Here's how the part is built. I have some questions about the finished solid (model axes, mm). Round coordinates to 2 decimals unless told otherwise and drop trailing zeros. Loops run counter-clockwise (first coordinate to the right, second up) from the corner with the lowest first, then second, coordinate; pieces in that order, holes last. Notation, with made-up numbers: M 66,55.25 L 80,55.25 A29 ccw 80,80.25 Z; hole C 13.25,55.25 d11. An arc over 180 degrees is marked long. Use a Markdown table: item, result.
```python
from build123d import *

# Parameters (mm, degrees)
SKETCH1_R           = 10.922
BOSS_EXTRUDE1_DEPTH = 5.08
SKETCH4_W           = 2.413
SKETCH4_H           = 2.413


with BuildPart() as part:
    # Sketch1 → Boss-Extrude1 (new body)
    with BuildSketch(Plane(origin=(0, 0, 0), x_dir=(1, 0, 0), z_dir=(0, 1, 0))):
        with Locations(Location((0, 0, 0), (0, 0, 270))):
            Circle(SKETCH1_R)
    extrude(amount=BOSS_EXTRUDE1_DEPTH)

    # Sketch4 → Cut-Revolve1 (revolve, cut)
    with BuildSketch(Plane.XY, mode=Mode.PRIVATE) as cut_revolve1_sk:
        with Locations((10.8077, 2.4765)):
            Rectangle(SKETCH4_W, SKETCH4_H)
    revolve(cut_revolve1_sk.sketch.rotate(Axis((0, 0, 0), (0, 1, 0)), 90), axis=Axis((0, 0, 0), (0, 1, 0)), mode=Mode.SUBTRACT)

    # Sketch5 → Revolve1 (revolve)
    with BuildSketch(Plane.XY, mode=Mode.PRIVATE) as revolve1_sk:
        with BuildLine():
            Line((10.16, 5.08), (2.600807741, 15.875645358))
            ThreePointArc((2.600807741, 15.875645358), (1.466051847, 16.870799568), (0, 17.229540172))
            Line((0, 17.229540172), (0, 5.08))
            Line((0, 5.08), (10.16, 5.08))
        make_face()
    revolve(revolve1_sk.sketch.rotate(Axis((0, 21.184130684, 0), (0, -1, 0)), 270), axis=Axis((0, 21.184130684, 0), (0, -1, 0)))


solid = part.part
```
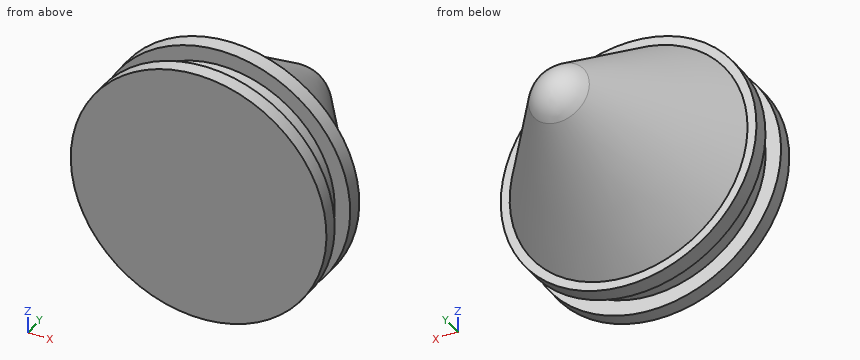
Q1. Imagine slicing it at A-A, the plane z = 0. Please give me the cut outline in (x, y) (3 decimals), then the cut area to 3 significant figures.
Return value:
| item | result |
|---|---|
| outline | M -10.922,0 L 10.922,0 L 10.922,1.27 L 9.601,1.27 L 9.601,3.683 L 10.922,3.683 L 10.922,5.08 L 10.16,5.08 L 2.601,15.876 A3.175 ccw -2.601,15.876 L -10.16,5.08 L -10.922,5.08 L -10.922,3.683 L -9.601,3.683 L -9.601,1.27 L -10.922,1.27 Z |
| area | 247 mm^2 |
Q2. Imagine slicing it at B-B, the plane x = 0. Please give me the cut outline in (y, z) (3 decimals).
Return value:
| item | result |
|---|---|
| outline | M 0,-10.922 L 1.27,-10.922 L 1.27,-9.601 L 3.683,-9.601 L 3.683,-10.922 L 5.08,-10.922 L 5.08,-10.16 L 15.876,-2.601 A3.175 ccw 15.876,2.601 L 5.08,10.16 L 5.08,10.922 L 3.683,10.922 L 3.683,9.601 L 1.27,9.601 L 1.27,10.922 L 0,10.922 Z |
Q3. Will these pins go through, and if not, where does the flat tip stop? P1, Ø1, axis at x = 6.5, z = -5.5, coming from the +Y side; P2, Ø2, axis at y = 5.5, z = -7, coming from the +X side; P3, Ø8, axis at y = 13.5, z = 4.5, coming from the +X side.
Return value:
| item | result |
|---|---|
| P1 | stops at y = 8.14 |
| P2 | stops at x = 9.06 |
| P3 | stops at x = 6.21 |
Q4. Imagine slicing it at D-D, the plane y = 8. Please give me the cut outline in (x, z), then the cut area to 3 significant figures.
Return value:
| item | result |
|---|---|
| outline | C 0,0 d16.23 |
| area | 207 mm^2 |
Q5. I need wall thicknesses on line 1 (Y direction, x = -6, z = 8.5); line 2 (X direction, y = 2.25, z = 5.75); line 3 (X direction, y = 12, z = 4). Which ranges of each line are inside material? Lowest first, please. Write a range as from..to.
Return value:
| item | result |
|---|---|
| line 1 | y = 0..1.27, 3.68..5.08 |
| line 2 | x = -7.69..7.69 |
| line 3 | x = -3.5..3.5 |
Q6. Imagine slicing it at C-C, the plane y = 4. Please give me the cut outline in (x, z).
Return value:
| item | result |
|---|---|
| outline | C 0,0 d21.84 |
